Autodesk Fusion 360 part; units mm, degrees
sketch "Sketch1" plane through (0, 0, 0) normal (0, 0, 1) x (1, 0, 0)
  line L0 (0, 0) -> (134, 0)
  line L1 (134, 0) -> (134, 183.541)
  line L2 (134, 183.541) -> (0, 183.541)
  line L3 (0, 183.541) -> (0, 0)
  circle A0 centre (7, 171.541) radius 1.55
  circle A1 centre (7, 12) radius 1.55
  circle A2 centre (7, 91.771) radius 1.55
  line L4 (67, 0) -> (67, 183.541) construction
  circle A3 centre (127, 12) radius 1.55
  circle A4 centre (127, 91.771) radius 1.55
  circle A5 centre (127, 171.541) radius 1.55
  line L5 (119.5, 174.041) -> (14.5, 174.041)
  line L6 (14.5, 174.041) -> (14.5, 169.041)
  line L7 (14.5, 169.041) -> (119.5, 169.041)
  line L8 (119.5, 169.041) -> (119.5, 174.041)
  line L9 (119.5, 174.041) -> (14.5, 169.041) construction
  line L10 (14.5, 174.041) -> (119.5, 169.041) construction
  line L11 (119.5, 9.5) -> (14.5, 9.5)
  line L12 (14.5, 9.5) -> (14.5, 14.5)
  line L13 (14.5, 14.5) -> (119.5, 14.5)
  line L14 (119.5, 14.5) -> (119.5, 9.5)
  line L15 (119.5, 9.5) -> (14.5, 14.5) construction
  line L16 (14.5, 9.5) -> (119.5, 14.5) construction
  line L17 (14.5, 9.5) -> (119.5, 174.041)
  line L18 (14.5, 14.5) -> (116.3093, 174.041)
  line L19 (119.5, 169.041) -> (17.6907, 9.5)
  line L20 (14.5, 174.041) -> (119.5, 9.5)
  line L21 (119.5, 14.5) -> (17.6907, 174.041)
  line L22 (14.5, 169.041) -> (116.3093, 9.5)
  point P0 (67, 171.541)
  point P1 (67, 12)
  dimension "d1" = 183.541
  dimension "d2" = 134
  dimension "d3" = 3.1
  dimension "d4" = 7
  dimension "d5" = 12
  dimension "d6" = 3.1
  dimension "d7" = 7
  dimension "d8" = 12
  dimension "d9" = 3.1
  dimension "d10" = 7
  dimension "d11" = 91.77
  dimension "d12" = 105
  dimension "d13" = 5
  dimension "d14" = 105
  dimension "d15" = 5
extrude "Extrude1" add sketch "Sketch1" along normal blind 1.5 contours L0 L1 L2 L3 | L5 L7 L17 L18 | L7 L8 L17 | L5 L7 L18 L21 | L7 L17 L19 L21 | L7 L17 L18 L21 | L5 L7 L20 L21 | L7 L18 L21 | L13 L19 L20 L21 | L17 L19 L20 L21 | L17 L18 L20 L21 | L6 L7 L20 | L7 L18 L20 L21 | L13 L19 L20 L22 | L17 L19 L20 L22 | L13 L14 L20 | L17 L18 L20 L22 | L7 L18 L20 L22 | L13 L19 L22 | L13 L17 L19 L22 | L11 L13 L20 L22 | L13 L17 L18 L22 | L11 L13 L17 L19 | L11 L13 L19 L22 | L12 L13 L17
extrude "Extrude2" add sketch "Sketch1" along normal blind 4 contours L5 L7 L17 L18 | L7 L8 L17 | L5 L7 L18 L21 | L7 L17 L19 L21 | L7 L17 L18 L21 | L5 L7 L20 L21 | L13 L19 L20 L21 | L17 L19 L20 L21 | L17 L18 L20 L21 | L6 L7 L20 | L7 L18 L20 L21 | L13 L19 L20 L22 | L17 L19 L20 L22 | L13 L14 L20 | L17 L18 L20 L22 | L7 L18 L20 L22 | L13 L17 L19 L22 | L11 L13 L20 L22 | L13 L17 L18 L22 | L11 L13 L17 L19 | L11 L13 L19 L22 | L12 L13 L17
equation "d6 = d3"
equation "d7 = d4"
equation "d8 = d5"
equation "d9 = d3"
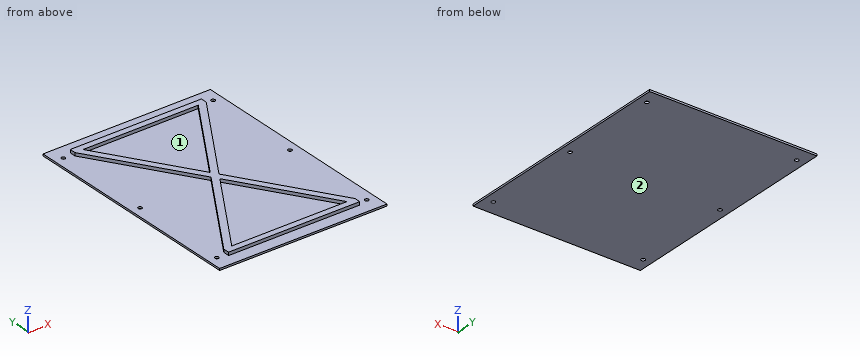
Part model, mm, in its own coordinate system. Face numbers are marked on the shaded views. Round coordinates to 2 decimals unless told otherwise and drop trailing zeros. Write each loop counter-clockwise with the first axis right and the second up, starting at its lowest first coordinate (ties: lowest second). Pieces come first, ordered by that corner, then holes.
Item 1: Cut at B-B, the plane x = 42. Give the cut face in (y, z), plus the area to 3 significant figures.
Results:
outline: (0, 0) - (183.54, 0) - (183.54, 1.5) - (174.04, 1.5) - (174.04, 4) - (169.04, 4) - (169.04, 1.5) - (135.95, 1.5) - (135.95, 4) - (125.95, 4) - (125.95, 1.5) - (57.59, 1.5) - (57.59, 4) - (47.59, 4) - (47.59, 1.5) - (14.5, 1.5) - (14.5, 4) - (9.5, 4) - (9.5, 1.5) - (0, 1.5) - close
area: 350 mm2
Item 2: Cut at A-A, the plane z = 2.9. Give the cut face in (x, y), plus the area to 3 significant figures.
Results:
outline: (14.5, 9.5) - (119.5, 9.5) - (119.5, 14.5) - (70.19, 91.77) - (119.5, 169.04) - (119.5, 174.04) - (14.5, 174.04) - (14.5, 169.04) - (63.81, 91.77) - (14.5, 14.5) - close; hole (20.88, 14.5) - (113.12, 14.5) - (67, 86.77) - close; hole (20.88, 169.04) - (67, 96.77) - (113.12, 169.04) - close
area: 2,990 mm2
Item 3: Probe L1, parallel to Y at x = 127, z = 0.6; L2, parallel to Y at x = 32, z = 3.6; L3, parallel to Z at x = 8, y = 116. List the from-to ranges inside material, lowest first.
Results:
L1: y = 0 to 10.45, 13.55 to 90.22, 93.32 to 169.99, 173.09 to 183.54
L2: y = 9.5 to 14.5, 31.92 to 41.92, 141.62 to 151.62, 169.04 to 174.04
L3: z = 0 to 1.5
Item 4: Drop flat-ended pins along their axis: pin 1 Ø0.8 at (y, z) = (12.5, 2) entering from -X; pin 2 Ø1.2 at (y, z) = (170.5, 2.5) entering from +X; pin 3 Ø5 at (x, y) = (127, 12) entering from +Z. Give the stop position or say it passes through.
Results:
pin 1: stops at x = 14.5
pin 2: stops at x = 119.5
pin 3: stops at z = 1.5
Item 5: Two-plate mould, pull along Y, no slides. Class the marked faces 1 and 2: +Y half, -Y half, draft (parallel to the pull), parting line (faces both ways), or undercut.
Results:
face 1: undercut
face 2: draft
Item 6: Cut at D-D, the plane x = 117. Give the cut face in (y, z).
Results:
outline: (0, 0) - (183.54, 0) - (183.54, 1.5) - (174.04, 1.5) - (174.04, 4) - (165.12, 4) - (165.12, 1.5) - (18.42, 1.5) - (18.42, 4) - (9.5, 4) - (9.5, 1.5) - (0, 1.5) - close
Item 7: Cut at C-C, the plane y = 106.5. Give the cut face in (x, z), plus the area to 3 significant figures.
Results:
outline: (0, 0) - (134, 0) - (134, 1.5) - (79.59, 1.5) - (79.59, 4) - (73.21, 4) - (73.21, 1.5) - (60.79, 1.5) - (60.79, 4) - (54.41, 4) - (54.41, 1.5) - (0, 1.5) - close
area: 233 mm2
